For this review, take the finished solid that the model builds, in its own axes (mm). A direction names the side the tool comes from. Coordinates: 2 decimals unless noted, no trailing zeros. Write each loop counter-clockwise with the first axis right and the second up, starting at its lowest first coordinate (ties: lowest second). Pieces come first, ordered by that corner, then holes. Notation, with made-up numbers: (88.5, 47) -> (112.5, 47) arc R24 ccw to (112.5, 68) -> close; hole circle Ø7 at (20.25, 16). An arc over 180 degrees is marked (long way). Put each result on its own line as item: value. Start each with the question number.
Item 1: For faces 5 (the flat face through (-30, 32, 57.5)), 6 (the cylindrical face through (-8.67, -39.05, 0.8)), 7 (the flat face through (-30, -30, 57.5)), list the 3-axis set-ups (+Z, -Z, +X, -X, +Y, -Y) from which the entire face can be reached by the end or side of a thin tool; tool diameter is ignored.
Item 2: The part is to be moulded in two halves that separate along X. For faces 1 (the flat face through (40, 1, 76)), 2 (the cylindrical face through (-30.925, 32.276, 76.259)), 3 (the cylindrical face through (-3.685, 1.596, 95.979)), 4 (the cylindrical face through (32.692, 30.793, 76.259)), say which applies: +X half, -X half, draft (parallel to the pull), parting line (faces both ways), or undercut.
Item 3: Consider section D-D on x = 11. Give the boundary of the cut face in (y, z), and give its area (3 significant figures).
Item 4: Consider section A-A on y = -15. Give the boundary of the cut face in (x, z), and give its area (3 significant figures).
Item 5: Insertion check: P1, Ø12, axis at x = 2, y = -29, coming from the +Z side; P2, Ø4, axis at x = 28, y = 11.5, coming from the +Z side; P3, Ø6, axis at y = -15, z = -30.5, coming from the +X side. Each pin has a flat end and moves straight along its axis. Give the tip position at first contact, or say it passes through.
Item 6: Consider section C-C on z = -10.5. Give the boundary of the cut face in (x, y).
Item 7: Consider section B-B on x = 29. Give the boundary of the cut face in (y, z).
Item 8: To check wall thickness, follow L1, parallel to Z at x = -25.5, y = -9.5; L2, parallel to Z at x = 31, y = -35; L3, parallel to Y at x = 0, z = -21. State the ranges of each line that lie inside material, in increasing order.
Autodesk Inventor part; units mm, degrees
ref_plane "YZ Plane" through (0, 0, 0) normal (1, 0, 0) x (0, 1, 0)
ref_plane "XZ Plane" through (0, 0, 0) normal (0, 1, 0) x (-1, 0, 0)
ref_plane "XY Plane" through (0, 0, 0) normal (0, 0, 1) x (1, 0, 0)
sketch "Sketch1" plane through (0, 0, 0) normal (0, 0, 1) x (1, 0, 0)
  circle A0 centre (0, 0) radius 40
  dimension "d0" = 80
extrude "Extrusion1" add sketch "Sketch1" along normal mid plane 115
sketch "Sketch3" plane through (0, 0, 57.5) normal (0, 0, 1) x (1, 0, 0)
  line L0 (-40, 40) -> (40, 40)
  line L1 (40, 40) -> (40, -40)
  line L2 (40, -40) -> (-40, -40)
  line L3 (-40, -40) -> (-40, 40)
  line L4 (-40, 40) -> (40, -40) construction
  line L5 (40, 40) -> (-40, -40) construction
  point P0 (0, 0)
  dimension "d9" = 80
  dimension "d10" = 80
extrude "Extrusion3" add sketch "Sketch3" along normal blind 37
sketch "Sketch4" plane through (0, 0, 94.5) normal (0, 0, 1) x (1, 0, 0)
  line L0 (0, 0) -> (0, -15)
  circle A0 centre (0, -15) radius 5
  dimension "d11" = 15
  dimension "d12" = 10
extrude "Extrusion4" add sketch "Sketch4" along normal blind 32
sketch "Sketch5" plane through (0, 0, 94.5) normal (0, 0, 1) x (1, 0, 0)
  circle A0 centre (0, -15) radius 17
  point P0 (0, 0)
  dimension "d15" = 34
extrude "Extrusion5" add sketch "Sketch5" along normal blind 3
sketch "Sketch6" plane through (0, 0, 94.5) normal (0, 0, 1) x (1, 0, 0)
  circle A0 centre (0, 0) radius 47
  line L0 (40, 0) -> (40, 40)
  line L1 (-40, 0) -> (-40, -40)
  line L2 (40, 40) -> (-40, -40)
  line L3 (-40, -40) -> (-40, 40)
  line L4 (40, -40) -> (40, 40)
  line L5 (-40, 40) -> (40, -40)
  circle A1 centre (33.234, 33.234) radius 2.5
  circle A2 centre (-33.234, 33.234) radius 2.5
  circle A3 centre (-33.234, -33.234) radius 2.5
  circle A4 centre (33.234, -33.234) radius 2.5
  dimension "d18" = 94
  dimension "d19" = 5
  dimension "d22" = 360
extrude "Extrusion6" cut sketch "Sketch6" against normal blind 40 contours A1 L2 A0 | A0 L2 A1 | A4 L5 A0 | A0 L5 A4 | L2 A1 A0 | A0 A1 L2 | L5 A4 A0 | A0 A4 L5 | A2 L5 A0 | A0 L5 A2 | A3 A0 L2 | L2 A0 A3 | A2 A0 L5 | A3 L2 A0 | A0 A2 L5 | L2 A3 A0
properties part number "MOTOR DC"
Return value:
1. face 5: -Z, -X, +Y
1. face 6: -Z
1. face 7: -Z, -X, -Y
2. face 1: +X half
2. face 2: undercut
2. face 3: parting line
2. face 4: undercut
3. outline: (-40, 57.5) -> (-38.46, 57.5) -> (-38.46, -57.5) -> (38.46, -57.5) -> (38.46, 57.5) -> (40, 57.5) -> (40, 94.5) -> (-2.04, 94.5) -> (-2.04, 97.5) -> (-27.96, 97.5) -> (-27.96, 94.5) -> (-40, 94.5) -> close
3. area: 11,900 mm^2
4. outline: (-40, 57.5) -> (-37.08, 57.5) -> (-37.08, -57.5) -> (37.08, -57.5) -> (37.08, 57.5) -> (40, 57.5) -> (40, 94.5) -> (17, 94.5) -> (17, 97.5) -> (5, 97.5) -> (5, 126.5) -> (-5, 126.5) -> (-5, 97.5) -> (-17, 97.5) -> (-17, 94.5) -> (-40, 94.5) -> close
4. area: 11,900 mm^2
5. P1: z = 97.5
5. P2: z = 94.5
5. P3: x = 38.16
6. outline: circle Ø80 at (0, 0)
7. outline: (-40, 57.5) -> (-27.55, 57.5) -> (-27.55, -57.5) -> (27.55, -57.5) -> (27.55, 57.5) -> (40, 57.5) -> (40, 94.5) -> (-40, 94.5) -> close
8. L1: -57.5 to 94.5
8. L2: 57.5 to 94.5
8. L3: -40 to 40
